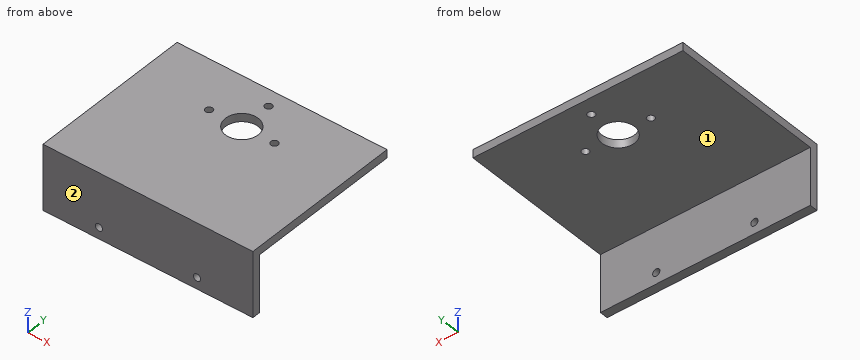
```python
from build123d import *

# Parameters (mm, degrees)
SKETCH1_W           = 81.531554226
SKETCH1_H           = 63.5
SKETCH1_R           = 6.35
SKETCH1_R_2         = 1.397
BOSS_EXTRUDE1_DEPTH = 3.175
SKETCH2_W           = 81.531554226
SKETCH2_H           = 3.175
BOSS_EXTRUDE2_DEPTH = 22.225
SKETCH3_R           = 1.397
CUT_EXTRUDE1_DEPTH  = 3175


with BuildPart() as part:
    # Sketch1 → Boss-Extrude1 (new body)
    with BuildSketch(Plane.XY):
        with Locations((0, -12.7)):
            Rectangle(SKETCH1_W, SKETCH1_H)
        Circle(SKETCH1_R, mode=Mode.SUBTRACT)
        with Locations((0, 12.7)):
            Circle(SKETCH1_R_2, mode=Mode.SUBTRACT)
        with Locations((-12.7, 0)):
            Circle(SKETCH1_R_2, mode=Mode.SUBTRACT)
        with Locations((12.7, 0)):
            Circle(SKETCH1_R_2, mode=Mode.SUBTRACT)
    extrude(amount=BOSS_EXTRUDE1_DEPTH)

    # Sketch2 → Boss-Extrude2 (add)
    with BuildSketch(Plane(origin=(0, 0, 0), x_dir=(-1, 0, 0), z_dir=(0, 0, -1))):
        with Locations((0, -42.8625)):
            Rectangle(SKETCH2_W, SKETCH2_H)
    extrude(amount=BOSS_EXTRUDE2_DEPTH)

    # Sketch3 → Cut-Extrude1 (cut)
    with BuildSketch(Plane(origin=(0, -41.275, 0), x_dir=(1, 0, 0), z_dir=(0, 1, 0))):
        with Locations(Location((-19.05, 17.78, 0), (0, 0, 270))):
            Circle(SKETCH3_R)
        with Locations(Location((19.05, 17.78, 0), (0, 0, 270))):
            Circle(SKETCH3_R)
    extrude(amount=-CUT_EXTRUDE1_DEPTH, mode=Mode.SUBTRACT)


solid = part.part
```
Read the model definition and answer for the solid it produces. Units are mm, in the model's axes. Face numbers are marked on the shaded views. A direction names the side the tool comes from. Give positions to 0.01 mm unless a question says otherwise; leave off trailing zeros. Write each loop counter-clockwise with the first axis right and the second up, starting at its lowest first coordinate (ties: lowest second). Pieces come first, ordered by that corner, then holes. Notation, with made-up numbers: (11.5, 61.25) - (62.5, 61.25) arc R16 cw to (62.5, 71.25) - close; hole circle Ø8 at (49, -39.75). An arc over 180 degrees is marked (long way). Write item = value, one per line. Start each with the question number.
Item 1: Find the intervals of material crossed by probe 1 along X at (y, z) = (-43.8, -17.78); probe 2 along Y at (x, z) = (0, 2.1); probe 3 along Z at (x, y) = (-19, -43) (3 decimals), in increasing order. Write a range as [from, to].
Item 2: Find section D-D (x = 23.5). Give the vertices of the cut face in (y, z) (3 decimals), then the cut area to 3 significant figures.
Item 3: A tool of negligible diameter and unlimited length cuts with its end or side. For the marked faces 1 and 2, from which of +Z, -Z, +X, -X, +Y, -Y can it reach the whole face along a straight path? Write none if from no direction.
Item 4: Find section A-A (x = -19.05). Give the vertices of the cut face in (y, z) (3 decimals).
Item 5: Find section B-B (y = 0). Give the vertices of the cut face in (x, z) (3 decimals).
Item 6: Each of these flat-tipped pins is pushed along its axis until it touches: P1, Ø10, axis at x = 31, z = -18.5, coming from the +Y side (3 decimals); P2, Ø3, axis at x = 0, y = 12.7, coming from the -Z side. Where does it stop, or does it pass through?
Item 7: Find section C-C (y = 12.7). Give the vertices of the cut face in (x, z) (3 decimals), then the cut area to 3 significant figures.
Response:
q1.probe_1 = [-40.77, -20.45], [-17.65, 17.65], [20.45, 40.77]
q1.probe_2 = [-44.45, -6.35], [6.35, 11.3], [14.1, 19.05]
q1.probe_3 = [-22.225, -19.176], [-16.384, 3.175]
q2.outline = (-44.45, -22.225) - (-41.275, -22.225) - (-41.275, 0) - (19.05, 0) - (19.05, 3.175) - (-44.45, 3.175) - close
q2.area = 272 mm²
q3.face_1 = -Z, +X, -X, +Y
q3.face_2 = +Z, -Z, +X, -X, -Y
q4.outline = (-44.45, -22.225) - (-41.275, -22.225) - (-41.275, -19.177) - (-44.45, -19.177) - close; (-44.45, -16.383) - (-41.275, -16.383) - (-41.275, 0) - (19.05, 0) - (19.05, 3.175) - (-44.45, 3.175) - close
q5.outline = (-40.766, 0) - (-14.097, 0) - (-14.097, 3.175) - (-40.766, 3.175) - close; (-11.303, 0) - (-6.35, 0) - (-6.35, 3.175) - (-11.303, 3.175) - close; (6.35, 0) - (11.303, 0) - (11.303, 3.175) - (6.35, 3.175) - close; (14.097, 0) - (40.766, 0) - (40.766, 3.175) - (14.097, 3.175) - close
q6.P1 = -41.275
q6.P2 = 0
q7.outline = (-40.766, 0) - (-1.397, 0) - (-1.397, 3.175) - (-40.766, 3.175) - close; (1.397, 0) - (40.766, 0) - (40.766, 3.175) - (1.397, 3.175) - close
q7.area = 250 mm²
